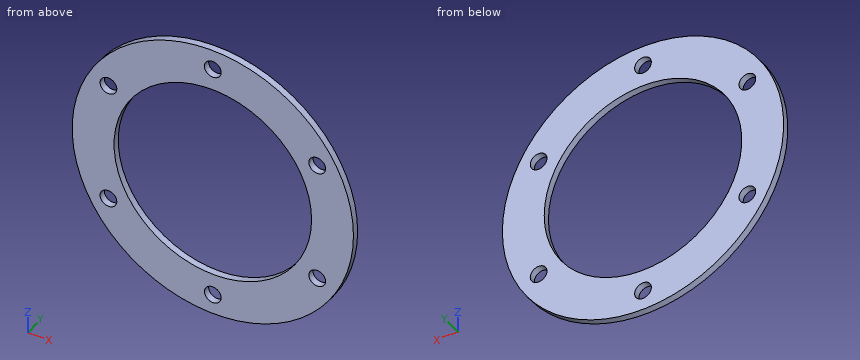
Solid Edge part; units mm, degrees
sketch "Sketch1" plane through (0, 0, 0) normal (0, -1, 0) x (1, 0, 0)
  circle A0 centre (0, 0) radius 42
extrude "Protrusion1" add sketch "Sketch1" along normal blind 2
sketch "Sketch2" plane through (0, -2, 0) normal (0, -1, 0) x (1, 0, 0)
  circle A0 centre (0, 0) radius 29.5
extrude "Cutout1" cut sketch "Sketch2" against normal through all
sketch "Sketch3" plane through (0, -2, 0) normal (0, -1, 0) x (1, 0, 0)
  circle A0 centre (0, 36) radius 2.5
extrude "Cutout2" cut sketch "Sketch3" against normal through all
pattern_circular "Pattern1" count 6 over 360 about axis through (0, -2, 0) along (0, 1, 0) of "Cutout2"
properties material "Aluminum, 1060"
The listing builds one solid part. Answer for the finished solid, in the listing's coordinates (mm). Round coordinates to 2 decimals unless told otherwise and drop trailing zeros. Order: outer loops, then holes, each group sorted by start corner. A loop starts at its lowest first (then second) coordinate and runs counter-clockwise, first axis right, second up. Notation, with made-up numbers: (51.25, -1) - (83.25, -1) arc R13 cw to (83.25, 4) - close; hole circle Ø2 at (86.5, 6). An arc over 180 degrees is marked (long way). Put each result on its own line as item: value. Start each with the question number.
(1) Find section C-C (x = 10). Give the vertices of the cut face in (y, z), plus the area to 3 significant figures.
(2) Find section B-B (x = 31). Give the vertices of the cut face in (y, z).
(3) Given P1, Ø1, axis at x = 25, z = 27.5, coming from the +Y side; P2, Ø4, axis at x = 31.18, z = -18, coming from the -Y side, each flat-ended and moving along its own axis, determine where each tip first touches the part or whether it passes through.
(4) Find section D-D (z = 18). Give the vertices of the cut face in (x, y).
(5) Straight lines are drawn through the part: probe 1 along Z at (x, y) = (-30, -0.1); probe 2 along Z at (x, y) = (30.5, -1.45); probe 3 along X at (y, z) = (-0.9, -19). For each, find the intervals that lie inside material, in ascending order. Write a range as from..to.
(6) Find section A-A (z = 0). Give the vertices of the cut face in (x, y).
Reply:
1. outline: (-2, -40.79) - (0, -40.79) - (0, -27.75) - (-2, -27.75) - close; (-2, 27.75) - (0, 27.75) - (0, 40.79) - (-2, 40.79) - close
1. area: 52.2 mm^2
2. outline: (-2, -28.34) - (0, -28.34) - (0, -20.49) - (-2, -20.49) - close; (-2, -15.51) - (0, -15.51) - (0, 15.51) - (-2, 15.51) - close; (-2, 20.49) - (0, 20.49) - (0, 28.34) - (-2, 28.34) - close
3. P1: y = 0
3. P2: through
4. outline: (-37.95, -2) - (-33.68, -2) - (-33.68, 0) - (-37.95, 0) - close; (-28.68, -2) - (-23.37, -2) - (-23.37, 0) - (-28.68, 0) - close; (23.37, -2) - (28.68, -2) - (28.68, 0) - (23.37, 0) - close; (33.68, -2) - (37.95, -2) - (37.95, 0) - (33.68, 0) - close
5. probe 1: -29.39..-20.21, -15.79..15.79, 20.21..29.39
5. probe 2: -28.87..-20.41, -15.59..15.59, 20.41..28.87
5. probe 3: -37.46..-33.47, -28.89..-22.57, 22.57..28.89, 33.47..37.46
6. outline: (-42, -2) - (-29.5, -2) - (-29.5, 0) - (-42, 0) - close; (29.5, -2) - (42, -2) - (42, 0) - (29.5, 0) - close
